Geometry: final body of the model. Coordinates: model frame, mm. A direction names the side the tool comes from. Round coordinates to 2 decimals unless told otherwise and drop trailing zeros. Write each loop counter-clockwise with the first axis right and the second up, starting at its lowest first coordinate (ties: lowest second). Pieces come first, ordered by that corner, then holes. Notation, with made-up numbers: M 86,41.25 L 141,41.25 A8 cw 141,52.25 Z; hole C 44.25,-34 d3. An arc over 180 degrees is marked long. Answer as CSV lines item,"result". Start each with the question number.
Q1. Mould query, pull axis Z, two halves, no side actions, for faces 4 (the cylindrical face through (-39.43, 0.6, 0.52)), 5 (the cylindrical face through (39.4, 15.82, -39.43)), 6 (the flat face through (-30, 16, -12.5)), 7 (the flat face through (-1, 16, 40)). Classes: pulls with the +Z half, pulls with the -Z half, needs draft (parallel to the pull), parting line crosses it, or undercut.
Q2. Section query A-A on x = 32. Output: boundary loops of the cut face in (y, z).
Q3. First-contact query: pin 1 (18 mm diameter, centred on y = 16, z = 25, fed in from -X). Flat tip, straight axial feed; report the tip coordinate or a pass-through.
Q4. Reachability of faces 1 (the flat face through (1, 0, 1)), 2 (the cylindrical face through (0.28, 8.137, -32.692)), 3 (the flat face through (-30, 25, 0)) from +Z, -Z, +X, -X, +Y, -Y: full face, straight path, thin tool, end or side. Return the list, or none.
Q5. Section query D-D on z = 18. Output: boundary loops of the cut face in (x, y).
Q6. Ray query, probe 1 along Z at (x, y) = (-32.25, 16); probe 2 along Y at (x, z) = (27, -25); probe 3 along Z at (x, y) = (-2.5, 16). Return the intervals inside material, ascending.
Q7. Section query B-B on z = -23.5. Output: boundary loops of the cut face in (x, y).
Autodesk Inventor part; units mm, degrees
ref_plane "YZ Plane" through (0, 0, 0) normal (1, 0, 0) x (0, 1, 0)
ref_plane "XZ Plane" through (0, 0, 0) normal (0, 1, 0) x (-1, 0, 0)
ref_plane "XY Plane" through (0, 0, 0) normal (0, 0, 1) x (1, 0, 0)
sketch "Sketch1" plane through (0, 0, 0) normal (0, 1, 0) x (-1, 0, 0)
  line L0 (40, 40) -> (-40, 40)
  line L1 (-40, 40) -> (-40, -40)
  line L2 (-40, -40) -> (40, -40)
  line L3 (40, -40) -> (40, 40)
  point P0 (0, 0)
  point P1 (40, 0)
  point P2 (0, 40)
  dimension "d0" = 80
  dimension "d1" = 80
extrude "Extrusion1" add sketch "Sketch1" along normal blind 32
sketch "Sketch27" plane through (-40, 0, 40) normal (0, 0, 1) x (1, 0, 0)
  line L0 (20, 27) -> (60, 27)
  line L1 (60, 27) -> (60, 5)
  line L2 (60, 5) -> (20, 5)
  line L3 (20, 5) -> (20, 27)
  line L4 (0, 0) -> (80, 0)
  line L5 (0, 32) -> (80, 32)
  line L6 (0, 0) -> (0, 32)
  line L7 (80, 0) -> (80, 32)
  point P0 (40, 0)
  dimension "d171" = 5
  dimension "d172" = 5
  dimension "d173" = 20
  dimension "d174" = 20
extrude "Extrusion21" cut sketch "Sketch27" against normal up to next contours L0 L1 L2 L3
sketch "Sketch28" plane through (-40, 0, -40) normal (-1, 0, 0) x (0, 0, 1)
  line L0 (0, 0) -> (0, 32)
  point P0 (40, 0)
  point P1 (15, 16)
  point P2 (65, 16)
  point P3 (0, 16)
  point P4 (0, 16)
  dimension "d177" = 25
  dimension "d178" = 25
hole "Hole8" at (-40, 16, -25) at (-40, 16, 25) direction (1, 0, 0) diameter 20 end through all
sketch "Sketch29" plane through (-40, 0, -40) normal (-1, 0, 0) x (0, 0, 1)
  line L0 (52.5, 25) -> (27.5, 25)
  line L1 (27.5, 25) -> (27.5, 7)
  line L2 (27.5, 7) -> (52.5, 7)
  line L3 (52.5, 7) -> (52.5, 25)
  line L4 (0, 32) -> (80, 32)
  line L5 (0, 0) -> (80, 0)
  point P0 (40, 0)
  point P1 (40, 7)
  point P2 (40, 0)
  dimension "d186" = 7
  dimension "d187" = 7
  dimension "d188" = 25
extrude "Extrusion22" cut sketch "Sketch29" against normal through all
extrude "Extrusion23" add sketch "Sketch27" against normal blind 4 contours L0 L1 L2 L3
sketch "Sketch30" plane through (40, 0, -40) normal (0, 0, -1) x (-1, 0, 0)
  line L0 (20, 27) -> (60, 27)
  line L1 (60, 5) -> (20, 5)
  line L2 (20, 5) -> (20, 27)
  line L3 (20, 27) -> (60, 27)
  line L4 (60, 27) -> (60, 5)
  point P0 (40, 0)
extrude "Extrusion24" add sketch "Sketch30" against normal blind 4
fillet "Fillet23" radius 11 4 edges at (0, 5, -36) (0, 27, -36) (0, 27, 36) (0, 5, 36)
fillet "Fillet24" radius 3 4 edges at (0, 32, 40) (0, 0, 40) (0, 32, -40) (0, 0, -40)
fillet "Fillet25" radius 2 16 edges at (40, 31.1213, -39.1213) (40, 16, -40) (40, 0.8787, -39.1213) (40, 0, 0) (40, 0.8787, 39.1213) (40, 16, 40) (40, 31.1213, 39.1213) (40, 32, 0) (-40, 31.1213, 39.1213) (-40, 16, 40) (-40, 0.8787, 39.1213) (-40, 0, 0) (-40, 0.8787, -39.1213) (-40, 16, -40) (-40, 31.1213, -39.1213) (-40, 32, 0)
properties part number "Y_Slider_Part_mit_Schrittmotor"
Entries:
1,face 4,"needs draft"
1,face 5,"pulls with the -Z half"
1,face 6,"undercut"
1,face 7,"pulls with the +Z half"
2,outline,"M 0,-37 A3 ccw 3,-40 L 29,-40 A3 ccw 32,-37 L 32,37 A3 ccw 29,40 L 3,40 A3 ccw 0,37 Z; hole C 16,-25 d20; hole C 16,25 d20; hole M 7,-12.5 L 25,-12.5 L 25,12.5 L 7,12.5 Z"
3,pin 1,"passes through"
4,face 1,"+Z, -Z, +X, -X, -Y"
4,face 2,"none"
4,face 3,"+X, -X"
5,outline,"M -40,2 A2 ccw -38,0 L 38,0 A2 ccw 40,2 L 40,8.86 L 20,8.86 L 20,5 L -20,5 L -20,8.86 L -40,8.86 Z; M -40,23.14 L -20,23.14 L -20,27 L 20,27 L 20,23.14 L 40,23.14 L 40,30 A2 ccw 38,32 L -38,32 A2 ccw -40,30 Z"
6,probe 1,"z = -40 to -35, -15 to -12.5, 12.5 to 15, 35 to 40"
6,probe 2,"y = 0 to 6, 26 to 32"
6,probe 3,"z = -40 to -36, 36 to 40"
7,outline,"M -40,2 A2 ccw -38,0 L 38,0 A2 ccw 40,2 L 40,6.11 L 20,6.11 L 20,5 L -20,5 L -20,6.11 L -40,6.11 Z; M -40,25.89 L -20,25.89 L -20,27 L 20,27 L 20,25.89 L 40,25.89 L 40,30 A2 ccw 38,32 L -38,32 A2 ccw -40,30 Z"
